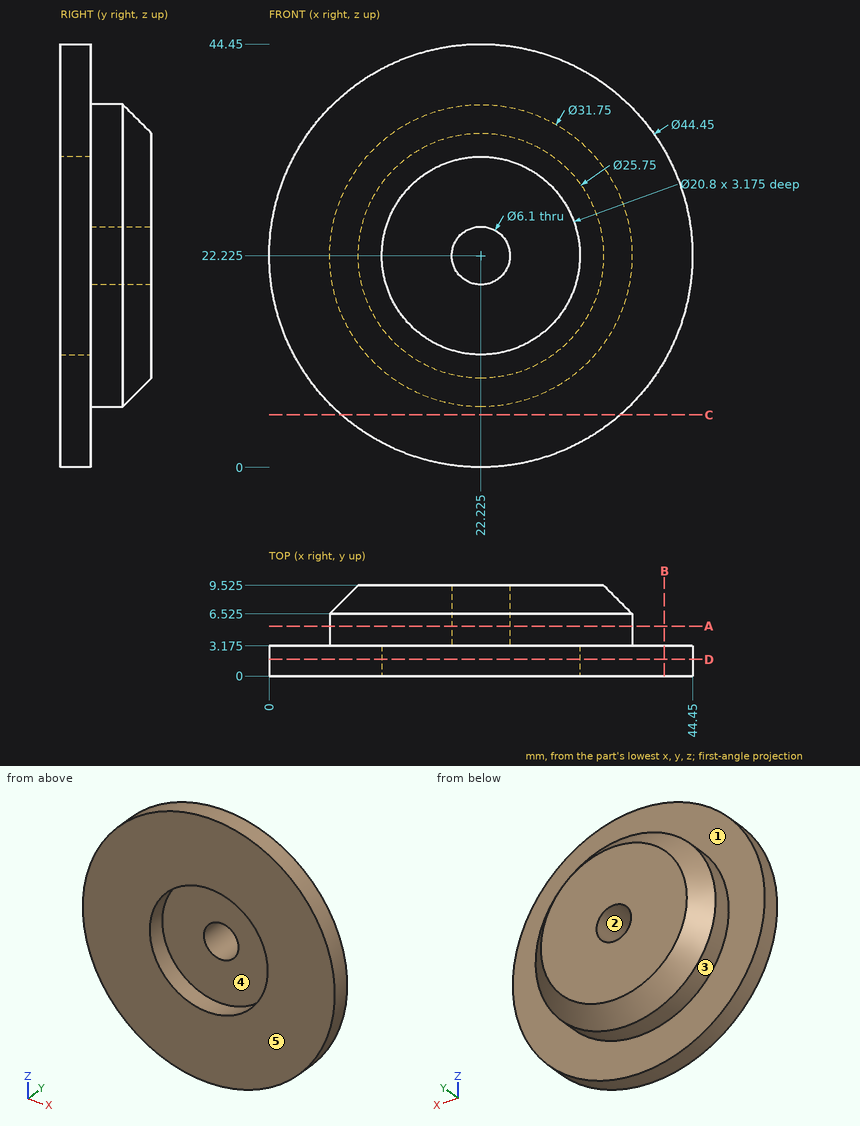
Input: dimensioned drawing with shaded views. Units: mm. Origin: part minimum x, y, z. A direction names the side the tool comes from. Coordinates: 2 decimals unless noted, no trailing zeros. Order: outer loops, then holes, each group sorted by start corner. A loop starts at its lowest first (then second) coordinate and runs counter-clockwise, first axis right, second up.
(1) Section query C-C (z = 5.5). Return the cut outline in (x, y) (3 decimals).
(2) Material intervals for probe 1 along Z at (x, y) = (22.5, 4.5); probe 2 along Y at (x, z) = (7, 6.5) (3 decimals); probe 3 along Y at (x, z) = (13.5, 26) (3 decimals), sorted ascending.
(3) Access query for the marked faces 4 and 5. Directions: +Z, -Z, +X, -X, +Y, -Y. A direction counts if a zero-diameter tool reaches every point of the face in a straight line with its end or side. Return the directions, or none.
(4) First-contact query: pin 1 (3 mm diameter, centred on x = 33, y = 5, fed in from -Z); pin 2 (4 mm diameter, centred on x = 20, y = 1.5, fed in from -Z); pin 3 (4 mm diameter, centred on y = 8, z = 23, fed in from +X). Flat tips, straight axial feed; report the tip coordinate or a pass-through.
(5) Section query D-D (y = 1.75). Return the cut outline in (x, z) (3 decimals).
(6) Draft query along Z for the marked faces 1, 2 and 3. Return one class per face: pulls with the +Z half, pulls with the -Z half, needs draft (parallel to the pull), parting line crosses it, or undercut.
(7) Section query B-B (x = 41.5). Return the cut outline in (y, z) (3 decimals).
(8) Section query A-A (y = 5.25). Return the cut outline in (x, z) (3 decimals).
Solution:
1. outline: (7.589, 0) - (36.861, 0) - (36.861, 3.175) - (7.589, 3.175) - close
2. probe 1: z = 6.35 to 19.19, 25.26 to 38.1
2. probe 2: y = 0 to 3.175
2. probe 3: y = 3.175 to 9.525
3. face 4: -Y
3. face 5: +Z, -Z, +X, -X, -Y
4. pin 1: stops at z = 9.34
4. pin 2: stops at z = 0
4. pin 3: stops at x = 38.1
5. outline: circle Ø44.45 at (22.225, 22.225); hole circle Ø20.8 at (22.225, 22.225)
6. face 1: needs draft
6. face 2: undercut
6. face 3: parting line crosses it
7. outline: (0, 11.16) - (3.175, 11.16) - (3.175, 33.29) - (0, 33.29) - close
8. outline: circle Ø31.75 at (22.225, 22.225); hole circle Ø6.1 at (22.225, 22.225)
